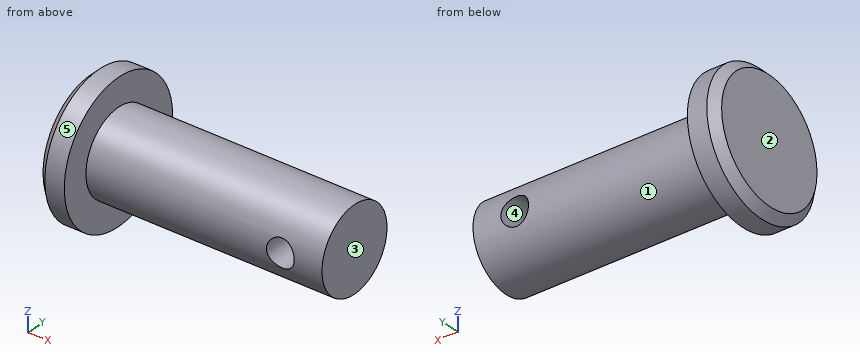
Autodesk Inventor part; units mm, degrees
ref_plane "Arbeitsebene1" through (5.25, 1.5, 0) normal (0, 1, 0) x (-1, 0, 0)
ref_plane "YZ Plane" through (0, 0, 0) normal (1, 0, 0) x (0, 1, 0)
ref_plane "XY Plane" through (0, 0, 0) normal (0, 0, 1) x (1, 0, 0)
sketch "Skizze1" plane through (0, 0, 0) normal (0, 0, 1) x (1, 0, 0)
  line L0 (0, -0.5) -> (0, 3)
  line L1 (-1.9, 0) -> (11.4, 0)
  line L2 (0, 0) -> (0, 2.5)
  line L3 (1, 2.5) -> (1, 1.5)
  line L4 (1, 1.5) -> (9.5, 1.5)
  line L5 (9.5, 1.5) -> (9.5, 0)
  line L6 (0, 0) -> (9.5, 0)
  line L7 (0, 2.5) -> (1, 2.5)
  dimension "d0" = 5
  dimension "d1" = 3
  dimension "d2" = 9.5
  dimension "d3" = 8.5
revolve "Umdrehung1" add sketch "Skizze1" angle 360 about axis through (-10, 0, 0) along (1, 0, 0)
chamfer "Fase1" distance 0.3 angle 45 1 edges at (0, -2.5, 0)
ref_plane "Arbeitsebene1" through (5.25, 1.5, 0) normal (0, 1, 0) x (-1, 0, 0)
sketch "Skizze2" plane through (5.25, 1.5, 0) normal (0, 1, 0) x (-1, 0, 0)
  line L0 (4.25, 1.5) -> (4.25, -1.5)
  line L1 (-4.25, 1.5) -> (-4.25, -1.5)
  line L2 (4.25, 1.5) -> (4.25, -1.5)
  line L3 (-4.25, 1.5) -> (-4.25, -1.5)
  line L4 (4.25, 1.5) -> (-4.25, 1.5)
  line L5 (4.25, -1.5) -> (-4.25, -1.5)
  point P0 (5.25, 0)
  point P1 (-2.75, 0)
  dimension "d8" = 1.5
  dimension "d9" = 1.5
hole "Bohrung1" at (8, 1.5, 0) direction (0, -1, 0) diameter 1 end through all
properties part number "Bolzen"
For this review, take the finished solid that the model builds, in its own axes (mm). Face numbers are marked on the shaded views. A direction names the side the tool comes from. Round coordinates to 2 decimals unless told otherwise and drop trailing zeros. Loops run counter-clockwise (first coordinate to the right, second up) from the corner with the lowest first, then second, coordinate; pieces in that order, holes last.
Q1. Add section C-C on x = 8. Write out the cut boundary in (y, z).
Result sheet:
outline: (-1.41, -0.5) arc R1.5 ccw to (1.41, -0.5) - close; (-1.41, 0.5) - (1.41, 0.5) arc R1.5 ccw to start
Q2. Add section B-B on z = 0. Write out the cut boundary in (x, y).
Result sheet:
outline: (0, -2.2) - (0.3, -2.5) - (1, -2.5) - (1, -1.5) - (7.5, -1.5) - (7.5, 1.5) - (1, 1.5) - (1, 2.5) - (0.3, 2.5) - (0, 2.2) - close; (8.5, -1.5) - (9.5, -1.5) - (9.5, 1.5) - (8.5, 1.5) - close
Q3. Mouldability with a two-part tool opening along X and no side actions: class the marked faces 3, 4 and 5 as +X half, -X half, draft (parallel to the pull), parting line (faces both ways), or undercut.
Result sheet:
face 3: +X half
face 4: undercut
face 5: draft
Q4. To check wall thickness, follow line 1 along X through (y, z) = (0.3, 0); line 2 along X through (y, z) = (-1.6, 0.2); line 3 along Y through (x, z) = (3.75, -0.05). State the ranges of each line that lie inside material, in increasing order.
Result sheet:
line 1: x = 0 to 7.5, 8.5 to 9.5
line 2: x = 0 to 1
line 3: y = -1.5 to 1.5
Q5. Machinability: for the marked faces 1 and 2, which of the approach directions +Z, -Z, +X, -X, +Y, -Y give a long, thin tool a straight path to every point of the face, cutting with its end or side? Answer none if there is none.
Result sheet:
face 1: +X
face 2: +Z, -Z, -X, +Y, -Y
Q6. Add section D-D on x = 0.5. Write out the cut boundary in (y, z).
Result sheet:
outline: circle Ø5 at (0, 0)
Q7. Add section A-A on y = 0. Write out the cut boundary in (x, z).
Result sheet:
outline: (0, -2.2) - (0.3, -2.5) - (1, -2.5) - (1, -1.5) - (9.5, -1.5) - (9.5, 1.5) - (1, 1.5) - (1, 2.5) - (0.3, 2.5) - (0, 2.2) - close; hole circle Ø1 at (8, 0)
Q8. Insertion check: pin 1 Ø1 at (x, z) = (6, -1) entering from +Y; pin 2 Ø1 at (x, y) = (2.5, -1.5) entering from +Z; pin 3 Ø1.5 at (x, z) = (5, 1) entering from -Y. Each pin has a flat end and moves straight along its axis. Give the tip position at first contact, or say it passes through.
Result sheet:
pin 1: stops at y = 1.41
pin 2: stops at z = 1.12
pin 3: stops at y = -1.48
